Could you check a few things on this model? Use its own coordinates, in mm. A direction names the side the tool comes from. Round coordinates to 2 decimals unless told otherwise and drop trailing zeros. Answer in a Markdown table with one row per item.
```python
from build123d import *

# Parameters (mm, degrees)
F0_W     = 80
F0_H     = 80
F1_DEPTH = 55
F2_SIZE2 = 20
F2_SIZE  = 20
F3_W     = 14
F3_H     = 24
F4_DEPTH = 35
F4_TAPER = -40
F5_W     = 15
F5_H     = 2.5
F5_H_2   = 5.2806121111
F6_DEPTH = 50
F7_DEPTH = 10
F8_DEPTH = 5


# Not quite as in the source:
# - a feature names something its author has since deleted; it is built from what else it names


with BuildPart() as f1:
    # F0 (on Top) → F1 (new body)
    with BuildSketch(Plane.XY):
        with Locations((3.4524537623, -3.0448271871)):
            Rectangle(F0_W, F0_H)
    extrude(amount=F1_DEPTH)

    # F2
    f2_edges = [f1.edges().sort_by_distance(p)[0] for p in [
        (43.452454, -3.044827, 55),
        (3.452454, 36.955173, 55),
        (-36.547546, -3.044827, 55),
        (3.452454, -43.044827, 55),
    ]]
    chamfer(f2_edges, length=F2_SIZE, length2=F2_SIZE2)

    # F3 (on face) → F4 (cut)
    with BuildSketch(Plane.XY.offset(55)):
        with Locations((3.4524537623, -3.0448271871)):
            Rectangle(F3_W, F3_H)
    extrude(amount=-F4_DEPTH, taper=F4_TAPER, mode=Mode.SUBTRACT)

    # F5 (on face) → F6 (cut)
    with BuildSketch(Plane.XZ.offset(43.0448271871)):
        with Locations((10.9524537623, 18.75)):
            Rectangle(F5_W, F5_H)
        with Locations((-4.0475462377, 18.75)):
            Rectangle(F5_W, F5_H)
        with Locations((-4.0475462377, 14.8596939445)):
            Rectangle(F5_W, F5_H_2)
        with Locations((10.9524537623, 14.8596939445)):
            Rectangle(F5_W, F5_H_2)
    extrude(amount=-F6_DEPTH, mode=Mode.SUBTRACT)

    # F7 (cut): a face of the model
    f7_faces = [f1.faces().sort_by_distance(p)[0] for p in [
        (3.4524537623, 35.8739389153, 20),
    ]]
    extrude(f7_faces, amount=-F7_DEPTH, mode=Mode.SUBTRACT)

    # F8 (cut): a face of the model
    f8_faces = [f1.faces().sort_by_distance(p)[0] for p in [
        (3.4524537623, -18.0448271871, 12.2193878889),
    ]]
    extrude(f8_faces, amount=-F8_DEPTH, mode=Mode.SUBTRACT)


solid = f1.part
```
1) Will these pins go through, and if not, where does the flat tip stop? P1, Ø1.5, axis at y = -28.5, z = 36.5, coming from the +X side; P2, Ø1.5, axis at x = 7.5, y = -6, coming from the +Z side; P3, Ø3, axis at x = 19, z = 39, coming from the -Y side.
Computed:
| item | result |
|---|---|
| P1 | stops at x = 42.7 |
| P2 | stops at z = 7.22 |
| P3 | stops at y = -40.54 |
2) I need wall thicknesses on line 1 (X direction, y = -18, z = 19); line 2 (Z direction, x = -20.5, y = 31.5); line 3 (Z direction, x = 20, y = 6). Which ranges of each line are inside material? Lowest first, please.
Computed:
| item | result |
|---|---|
| line 1 | x = -36.55 to -32.92, 39.82 to 43.45 |
| line 2 | z = 0 to 10, 28.13 to 40.46 |
| line 3 | z = 0 to 10, 43.62 to 55 |
3) Which directions (+Z, -Z, +X, -X, +Y, -Y) give clear straight access to the entire face, cutting with the end or side of a thin tool? Please do faces 4 (the face through (-32.916, -4, 15)), 5 (the face through (12, -3, 55)), 6 (the face through (18.452, -18, 9)).
Computed:
| item | result |
|---|---|
| face 4 | +Y, -Y |
| face 5 | +Z, +X, -X, +Y, -Y |
| face 6 | -Y |
4) If we mould it in two halves opening along Z, with no side actions, what happens to faces 1 (the face through (3, -2, 0)), 2 (the face through (3, 6.955, 9)), 3 (the face through (2.892, 29.037, 42.918))? For each: released by +Z, released by -Z, zero draft, split by the parting line, or undercut.
Computed:
| item | result |
|---|---|
| face 1 | released by -Z |
| face 2 | undercut |
| face 3 | released by +Z |
